Geometry: see drawing. Coordinates: mm, zero at the bounding-box minimum. A direction names the side the tool comes from. Give positions to 0.01 mm unless a question says otherwise; leave off trailing zeros. Loops run counter-clockwise (first coordinate to the right, second up) from the corner with the lowest first, then second, coordinate; pieces in that order, holes last. Notation, with made-up numbers: (-14, -19.75) - (19, -19.75) arc R17 ccw to (19, -12.75) - close; hole circle Ø2 at (60.25, 44). An arc over 180 degrees is marked (long way). One line per question, with ' | ' between items. Start each with the question number.
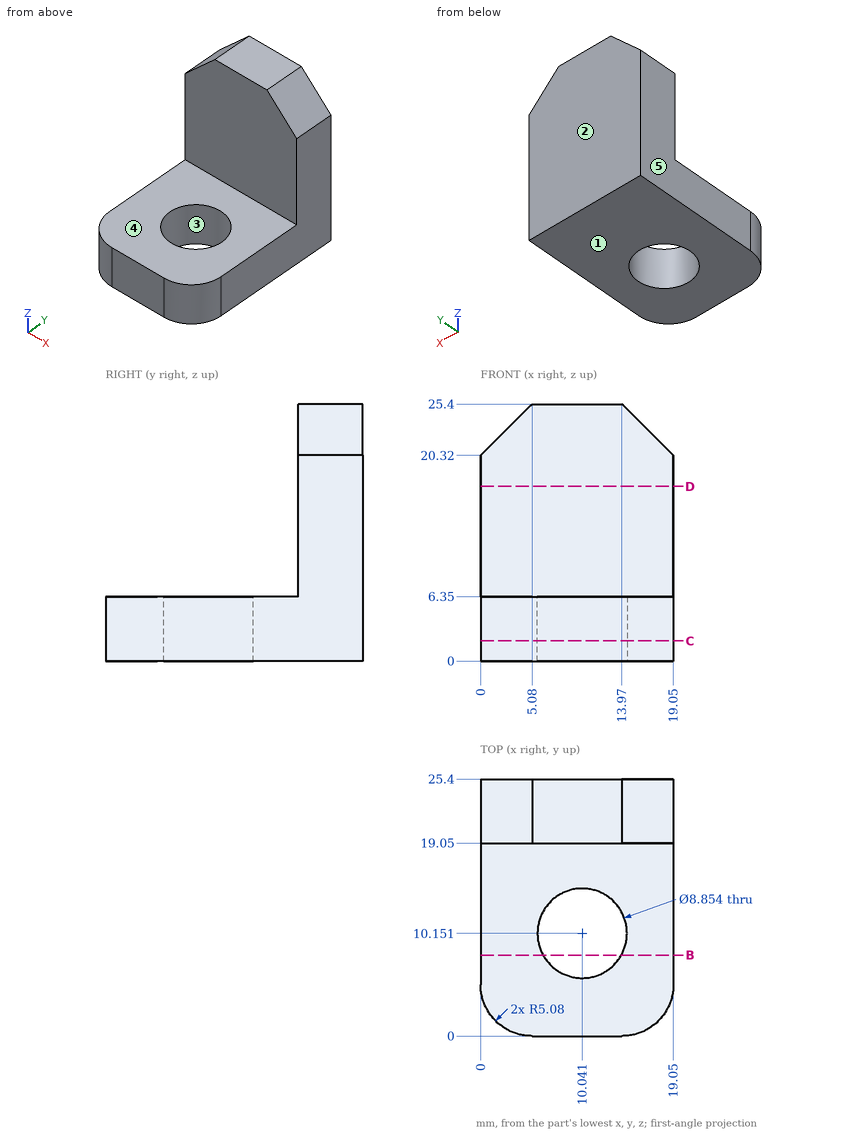
Q1. Access query for the marked faces 4 and 5. Directions: +Z, -Z, +X, -X, +Y, -Y. A direction counts if a zero-diameter tool reaches every point of the face in a straight line with its end or side. Return the directions, or none.
Q2. Section D-D, the plane z = 17.25. Output: boundary loops of the cut face in (x, y), plus the area to 3 significant figures.
Q3. First-contact query: pin 1 (5 mm diameter, centred on x = 13.5, z = 14.5, fed in from -Y); pin 2 (10 mm diameter, centred on x = 2.5, y = 22.5, fed in from -Z); pin 3 (1.5 mm diameter, centred on x = 8, y = 12, fed in from +Z). Flat tips, straight axial feed; report the tip coordinate or a pass-through.
Q4. Draft query along Y for the marked faces 1, 2 and 3. Return one class per face: +Y half, -Y half, draft (parallel to the pull), parting line (faces both ways), or undercut.
Q5. Section B-B, the plane y = 8. Output: boundary loops of the cut face in (x, z).
Q6. Section C-C, the plane z = 2. Output: boundary loops of the cut face in (x, y).
Q7. Line query: L1, parallel to Y at x = 10, z = 5.5; L2, parallel to Y at x = 7, z = 13.25; L3, parallel to Z at x = 2.5, y = 18. Output: solid intervals per line, ascending. Write a range as from..to.
Solved:
1) face 4: +Z, +X, -X, -Y | face 5: +Z, -Z, -X, +Y, -Y
2) outline: (0, 19.05) - (19.05, 19.05) - (19.05, 25.4) - (0, 25.4) - close | area: 121 mm²
3) pin 1: stops at y = 19.05 | pin 2: stops at z = 0 | pin 3: passes through
4) face 1: draft | face 2: +Y half | face 3: undercut
5) outline: (0, 0) - (6.17, 0) - (6.17, 6.35) - (0, 6.35) - close; (13.91, 0) - (19.05, 0) - (19.05, 6.35) - (13.91, 6.35) - close
6) outline: (0, 5.08) arc R5.08 ccw to (5.08, 0) - (13.97, 0) arc R5.08 ccw to (19.05, 5.08) - (19.05, 25.4) - (0, 25.4) - close; hole circle Ø8.85 at (10.04, 10.15)
7) L1: y = 0..5.72, 14.58..25.4 | L2: y = 19.05..25.4 | L3: z = 0..6.35
